The listing builds one solid part. Answer for the finished solid, in the listing's coordinates (mm). Face numbers are marked on the shaded views. A direction names the side the tool comes from. Coordinates: 2 decimals unless noted, no trailing zeros. Loops run counter-clockwise (first coordinate to the right, second up) from the corner with the lowest first, then second, coordinate; pieces in that order, holes last. Notation, with made-up numbers: (53, 17) - (112, 17) arc R9 cw to (112, 21) - close; hole circle Ø10 at (-28.5, 59.5). An arc over 180 degrees is marked (long way). Write each question's results on one line, items separated by ' | '. Start each with the question number.
(1) Given pin 1 Ø0.8 at (y, z) = (-29.5, -149) entering from -X; pin 2 Ø1 at (y, z) = (-119.5, -68) entering from -X; pin 3 Ø3 at (x, z) = (131, -157.5) entering from -Y, each flat-ended and moving along its own axis, determine where each tip first touches the part or whether it passes through.
(2) Consider line 1 (Z direction, x = 168.5, y = -90); line 2 (X direction, y = -62, z = -131); line 3 (Y direction, x = 117.5, z = -177). Determine where each line is inside the solid, lowest interval first. Write a range as from..to.
(3) Find section A-A on y = -44.5. Determine the outline of the cut face in (x, z), then the cut area to 4 significant figures.
(4) For the marked faces 1 and 2, determine the directions among +Z, -Z, +X, -X, +Y, -Y from which every point of the face is accessible in a straight line to the end or side of a thin tool.
(5) Determine the mould class of the marked faces 3, 4, 5 and 6 for opening direction Z: released by +Z, released by -Z, zero draft, split by the parting line, or undercut.
(6) Find section B-B on z = -126.5. Determine the outline of the cut face in (x, y).
(7) Find section C-C on z = -206.5. Determine the outline of the cut face in (x, y).
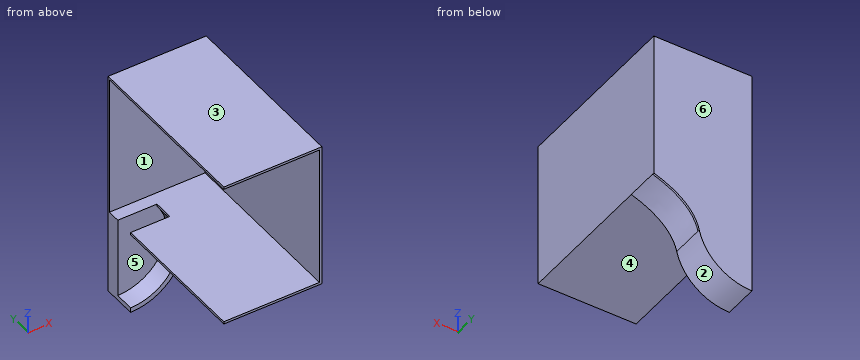
from build123d import *

# Parameters (mm, degrees)
BOX_W                                = 100
BOX_H                                = 200
BOX_DEPTH                            = 250
SKETCH004_W                          = 80
SKETCH004_H                          = 20
EXTRUDE005_DEPTH                     = 20
SKETCH_AS_DRAWN_W                    = 200
SKETCH_AS_DRAWN_H                    = 150
SKETCH_AS_DRAWN_W_2                  = 195
SKETCH_AS_DRAWN_H_2                  = 145
EXTRUDE_DEPTH                        = 180
EXTRUDE_ONTO_SKETCH_ROLL_ANGLE       = 90
EXTRUDE004_DEPTH                     = 20
EXTRUDE004_ONTO_SKETCH002_ROLL_ANGLE = 90
EXTRUDE002_DEPTH                     = 35
EXTRUDE002_ONTO_SKETCH003_ROLL_ANGLE = 90
EXTRUDE001_DEPTH                     = 2
EXTRUDE001_ONTO_SKETCH001_ROLL_ANGLE = 90


with BuildPart() as cube:
    # Box → Box (new body)
    with BuildSketch(Plane(origin=(0, -200, -240), x_dir=(1, 0, 0), z_dir=(0, 0, 1))):
        with Locations((50, 100)):
            Rectangle(BOX_W, BOX_H)
    extrude(amount=BOX_DEPTH)


with BuildPart() as extrude005:
    # Sketch004 → Extrude005 (new body)
    with BuildSketch(Plane.XY.offset(-147.5)):
        with Locations((100, -25)):
            Rectangle(SKETCH004_W, SKETCH004_H)
    extrude(amount=EXTRUDE005_DEPTH)


with BuildPart() as extrude005_1:
    # Extrude005 placement: moved
    add(extrude005.part.moved(Location((0, 0, -6))))


with BuildPart() as cut001:
    # Sketch as drawn → Extrude (new)
    with BuildSketch(Plane.XY):
        with Locations((100, -75)):
            Rectangle(SKETCH_AS_DRAWN_W, SKETCH_AS_DRAWN_H)
        with Locations((100, -75)):
            Rectangle(SKETCH_AS_DRAWN_W_2, SKETCH_AS_DRAWN_H_2, mode=Mode.SUBTRACT)
    extrude(amount=EXTRUDE_DEPTH)


with BuildPart() as cut001_1:
    # Extrude onto Sketch roll: moved
    add(cut001.part.rotate(Axis((0, 0, 0), (1, 0, 0)), EXTRUDE_ONTO_SKETCH_ROLL_ANGLE))


with BuildPart() as cut001_2:
    # Extrude onto Sketch placement: moved
    add(cut001_1.part)

    # Cut001: cut Extrude005
    add(extrude005_1.part, mode=Mode.SUBTRACT)


with BuildPart() as extrude004:
    # Sketch002 as drawn → Extrude004 (new)
    with BuildSketch(Plane.XY):
        with BuildLine():
            ThreePointArc((60, -150), (100, -230), (140, -150))
            Line((60, -150), (140, -150))
        make_face()
    extrude(amount=EXTRUDE004_DEPTH)


with BuildPart() as extrude004_1:
    # Extrude004 onto Sketch002 roll: moved
    add(extrude004.part.rotate(Axis((0, 0, 0), (1, 0, 0)), EXTRUDE004_ONTO_SKETCH002_ROLL_ANGLE))


with BuildPart() as extrude004_2:
    # Extrude004 onto Sketch002 placement: moved
    add(extrude004_1.part)


with BuildPart() as extrude004_3:
    # Extrude004 placement: moved
    add(extrude004_2.part.moved(Location((0, -15, 0))))


with BuildPart() as cut:
    # Sketch003 as drawn → Extrude002 (new)
    with BuildSketch(Plane.XY):
        with BuildLine():
            add(Edge.make_bspline(
                [(46.325052, -192), (40, -164), (0, -150)],
                knots=[0, 0, 0, 1, 1, 1], degree=2))
            Line((0, -150), (200, -150))
            add(Edge.make_bspline(
                [(200, -150), (160, -164), (153.674948, -192)],
                knots=[0, 0, 0, 1, 1, 1], degree=2))
            ThreePointArc((153.674948, -192), (100, -235), (46.325052, -192))
        make_face()
    extrude(amount=EXTRUDE002_DEPTH)


with BuildPart() as cut_1:
    # Extrude002 onto Sketch003 roll: moved
    add(cut.part.rotate(Axis((0, 0, 0), (1, 0, 0)), EXTRUDE002_ONTO_SKETCH003_ROLL_ANGLE))


with BuildPart() as cut_2:
    # Extrude002 onto Sketch003 placement: moved
    add(cut_1.part)

    # Cut: cut Extrude004
    add(extrude004_3.part, mode=Mode.SUBTRACT)


with BuildPart() as cut010:
    # Sketch001 as drawn → Extrude001 (new)
    with BuildSketch(Plane.XY):
        with BuildLine():
            add(Edge.make_bspline(
                [(46.325052, -192), (40, -164), (0, -150)],
                knots=[0, 0, 0, 1, 1, 1], degree=2))
            Line((0, -150), (0, 0))
            Line((0, 0), (200, 0))
            Line((200, 0), (200, -150))
            add(Edge.make_bspline(
                [(200, -150), (160, -164), (153.674948, -192)],
                knots=[0, 0, 0, 1, 1, 1], degree=2))
            ThreePointArc((153.674948, -192), (100, -235), (46.325052, -192))
        make_face()
    extrude(amount=EXTRUDE001_DEPTH)


with BuildPart() as cut010_1:
    # Extrude001 onto Sketch001 roll: moved
    add(cut010.part.rotate(Axis((0, 0, 0), (1, 0, 0)), EXTRUDE001_ONTO_SKETCH001_ROLL_ANGLE))


with BuildPart() as cut010_2:
    # Extrude001 onto Sketch001 placement: moved
    add(cut010_1.part)

    # Fusion: union Cut001, Cut
    add(cut001_2.part)
    add(cut_2.part)

    # Cut010: cut Cube
    add(cube.part, mode=Mode.SUBTRACT)


solid = cut010_2.part
Values:
1) pin 1: stops at x = 140 | pin 2: stops at x = 197.5 | pin 3: stops at y = -15
2) line 1: z = -150..-147.5, -2.5..0 | line 2: x = 197.5..200 | line 3: y = -15..0
3) outline: (100, -150) - (200, -150) - (200, 0) - (100, 0) - (100, -2.5) - (197.5, -2.5) - (197.5, -147.5) - (100, -147.5) - close | area: 862.5 mm²
4) face 1: -X, -Y | face 2: -Z, +X, +Y, -Y
5) face 3: released by +Z | face 4: released by -Z | face 5: undercut | face 6: zero draft
6) outline: (100, -2) - (197.5, -2) - (197.5, -180) - (200, -180) - (200, 0) - (100, 0) - close
7) outline: (100, -15) - (142.4, -15) - (142.4, -35) - (148.19, -35) - (148.19, 0) - (100, 0) - close
